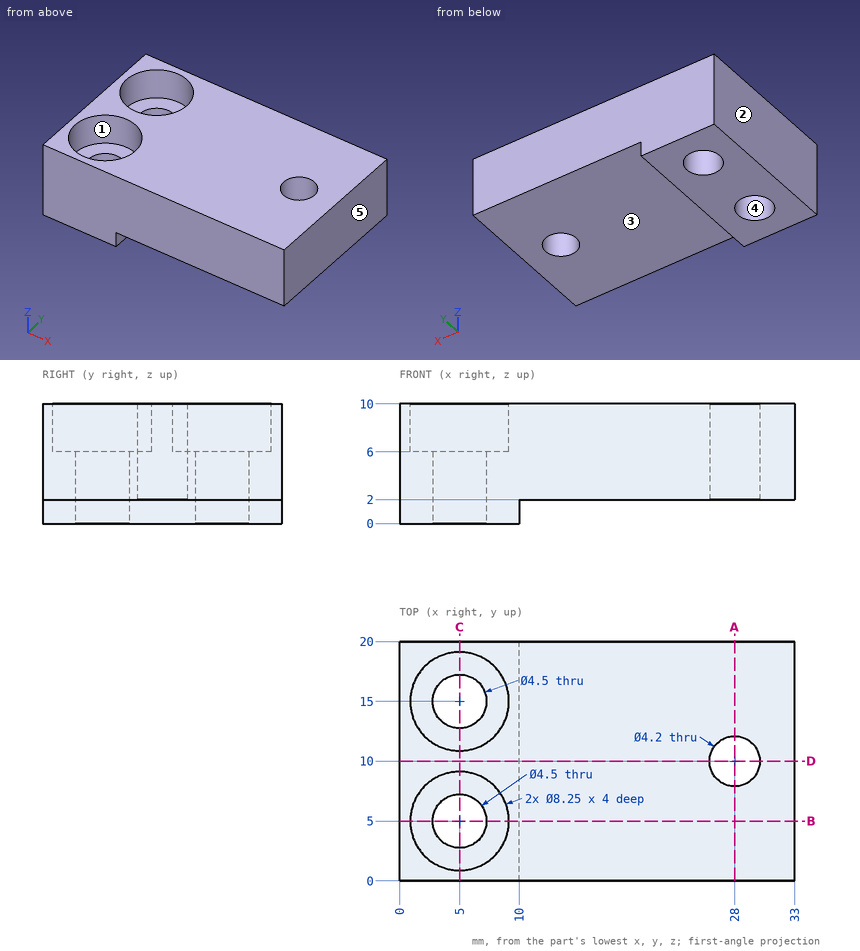
Geometry check sheet. Reference: drawing and pictorial views, mm from the part's lowest x, y, z. A direction names the side the tool comes from. Coordinates: 2 decimals unless noted, no trailing zeros. Write each loop counter-clockwise with the first axis right and the second up, starting at its lowest first coordinate (ties: lowest second). Pieces come first, ordered by that corner, then holes. Notation, with made-up numbers: M 70.5,11 L 106.5,11 A24 ccw 106.5,49 Z; hole C 75.25,18.5 d11. An arc over 180 degrees is marked long. Use one line per item in the form item = value.
Item 1: Release check for a two-part mould opening along X. For the marked faces 3, 4 and 5 record: pulls with the +X half, pulls with the -X half, needs draft (parallel to the pull), parting line crosses it, or undercut.
Answer below:
face_3 = needs draft
face_4 = undercut
face_5 = pulls with the +X half
Item 2: Gauge pin test, flat end, axial feed: pin 1 Ø5 at (x, y) = (5, 15) entering from +Z. Record the tip position at first contact, or that the pin passes through.
Answer below:
pin_1 = 6
Item 3: Sectioned sample at B-B, the plane y = 5. Record the cut outline in (x, z) (3 decimals).
Answer below:
outline = M 0,0 L 2.75,0 L 2.75,6 L 0.875,6 L 0.875,10 L 0,10 Z; M 7.25,0 L 10,0 L 10,2 L 33,2 L 33,10 L 9.125,10 L 9.125,6 L 7.25,6 Z
Item 4: Sectioned sample at C-C, the plane x = 5. Record the cut outline in (y, z) (3 decimals).
Answer below:
outline = M 0,0 L 2.75,0 L 2.75,6 L 0.875,6 L 0.875,10 L 0,10 Z; M 7.25,0 L 12.75,0 L 12.75,6 L 10.875,6 L 10.875,10 L 9.125,10 L 9.125,6 L 7.25,6 Z; M 17.25,0 L 20,0 L 20,10 L 19.125,10 L 19.125,6 L 17.25,6 Z
Item 5: Set-up check for the marked faces 1 and 2: record each of +Z, -Z, +X, -X, +Y, -Y from which the full face is reachable in a straight line by a thin tool's end or side.
Answer below:
face_1 = +Z
face_2 = +Z, -Z, -X, +Y, -Y
Item 6: Sectioned sample at A-A, the plane x = 28. Record the cut outline in (y, z), and give its area (3 significant figures).
Answer below:
outline = M 0,2 L 7.9,2 L 7.9,10 L 0,10 Z; M 12.1,2 L 20,2 L 20,10 L 12.1,10 Z
area = 126 mm^2
Item 7: Sectioned sample at D-D, the plane y = 10. Record the cut outline in (x, z), and give its area (3 significant figures).
Answer below:
outline = M 0,0 L 10,0 L 10,2 L 25.9,2 L 25.9,10 L 0,10 Z; M 30.1,2 L 33,2 L 33,10 L 30.1,10 Z
area = 250 mm^2
Item 8: Material ranges on L1, parallel to Y at x = 5, z = 1.55; L2, parallel to Y at x = 5, z = 7.5 (3 decimals); L3, parallel to X at y = 11.25, z = 8.5, recorded low to high. Write a range as from..to.
Answer below:
L1 = 0..2.75, 7.25..12.75, 17.25..20
L2 = 0..0.875, 9.125..10.875, 19.125..20
L3 = 0..3.28, 6.72..26.31, 29.69..33
